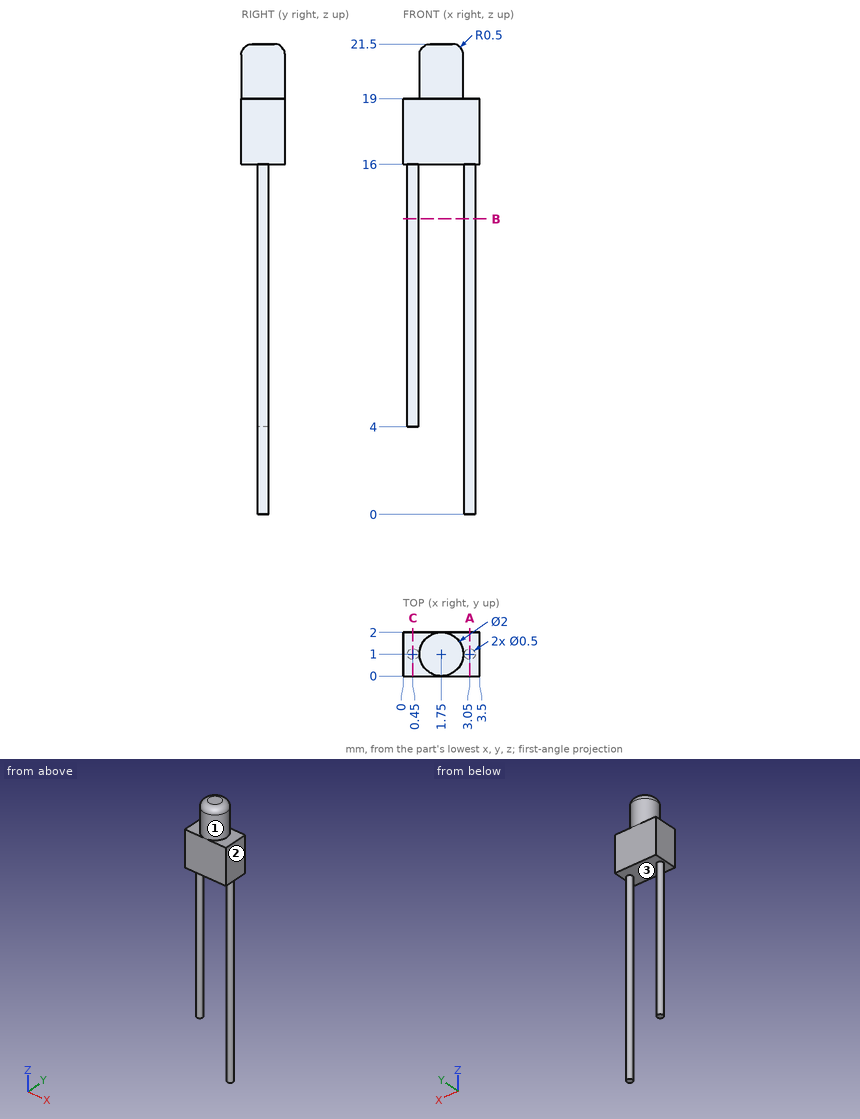
Design review of the part shown in the three views and the two pictorial views. Dimensions are in mm from the part's minimum x, y and z. A direction names the side the tool comes from. Coordinates: 2 decimals unless noted, no trailing zeros. Loops run counter-clockwise (first coordinate to the right, second up) from the corner with the lowest first, then second, coordinate; pieces in that order, holes last. Notation, with made-up numbers: (-19.75, -5.75) - (-6.75, -5.75) arc R18 ccw to (-6.75, 16.25) - close; hole circle Ø4 at (-28.75, 24.25). An arc over 180 degrees is marked (long way). Use a Markdown table: item, result. Add a question column.
Item 1: We need section A-A (x = 3.05). Give the boundary of the cut face in (y, z).
Item 2: For line 1 (X direction, y = 0.95, z = 7.5); line 2 (Z direction, x = 0.5, y = 1.45); line 3 (Z direction, x = 2.05, y = 0.55), list the stretches that pass through material, from the lowest coordinate up.
Item 3: Tool access review of the marked faces 1, 2 and 3: name each direction out of +Z, -Z, +X, -X, +Y, -Y from which nothing blocks a thin tool from reaching the whole face with its end or side.
Item 4: We need section C-C (x = 0.45). Give the boundary of the cut face in (y, z).
Item 5: We need section B-B (z = 13.5). Give the boundary of the cut face in (x, y), and give its area (3 significant figures).
Results list:
| question | item | result |
|---|---|---|
| 1 | outline | (0, 16) - (0.75, 16) - (0.75, 0) - (1.25, 0) - (1.25, 16) - (2, 16) - (2, 19) - (0, 19) - close |
| 2 | line 1 | x = 0.21 to 0.69, 2.81 to 3.29 |
| 2 | line 2 | z = 16 to 19 |
| 2 | line 3 | z = 16 to 21.5 |
| 3 | face 1 | +Z |
| 3 | face 2 | +Z, -Z, +X, +Y, -Y |
| 3 | face 3 | -Z |
| 4 | outline | (0, 16) - (0.75, 16) - (0.75, 4) - (1.25, 4) - (1.25, 16) - (2, 16) - (2, 19) - (0, 19) - close |
| 5 | outline | circle Ø0.5 at (0.45, 1); circle Ø0.5 at (3.05, 1) |
| 5 | area | 0.393 mm^2 |
